```python
from build123d import *

# Parameters (mm, degrees)
SKETCH1_R               = 50
BOSS_EXTRUDE1_DEPTH     = 5
BOSS_EXTRUDE3_START     = 5
BOSS_EXTRUDE3_DEPTH     = 5
DRAFT2_ANGLE            = -45
CUT_EXTRUDE3_DEPTH      = 72.414284285
CUT_EXTRUDE3_DEPTH_BACK = 72.414284285
SKETCH3_R               = 7.5
CUT_EXTRUDE5_START      = -6.666666667
CUT_EXTRUDE5_DEPTH      = 6.666666667
SKETCH5_R               = 3.55
SKETCH5_R_2             = 1.55
CUT_EXTRUDE6_DEPTH      = 72.414284285
SKETCH5_3_R             = 3.55
SKETCH5_3_R_2           = 1.55
BOSS_EXTRUDE4_DEPTH     = 2.5
CUT_EXTRUDE8_DEPTH      = 72.414284285
CHAMFER1_SIZE           = 5
CUT_EXTRUDE9_DEPTH      = 71.887234394


with BuildPart() as part:
    # Sketch1 → Boss-Extrude1 (new body)
    with BuildSketch(Plane(origin=(0, 0, 0), x_dir=(1, 0, 0), z_dir=(0, 1, 0))):
        with Locations(Location((0, 0, 0), (0, 0, 270))):
            Circle(SKETCH1_R)
    extrude(amount=-BOSS_EXTRUDE1_DEPTH)

    # Sketch1<6> → Boss-Extrude3 (add)
    with BuildSketch(Plane(origin=(0, 0, 0), x_dir=(1, 0, 0), z_dir=(0, 1, 0)).offset(BOSS_EXTRUDE3_START)):
        with BuildLine():
            Line((-12.940952256, 48.296291314), (-34.10533906, -36.562629112))
            ThreePointArc((-34.10533906, -36.562629112), (0, -50), (34.10533906, -36.562629112))
            Line((34.10533906, -36.562629112), (12.940952256, 48.296291314))
            ThreePointArc((12.940952256, 48.296291314), (0, 50), (-12.940952256, 48.296291314))
        make_face()
    extrude(amount=-BOSS_EXTRUDE3_DEPTH)

    # Draft2
    draft2_faces = [part.faces().sort_by_distance(p)[0] for p in [
        (23.523145658, 2.5, -5.866831101),
        (-23.523145658, 2.5, -5.866831101),
    ]]
    draft(draft2_faces, Plane.ZX, DRAFT2_ANGLE)

    # Sketch3 → Cut-Extrude3 (cut, two sides: drawn at the far end of the back side and taken through both)
    with BuildSketch(Plane.XZ.offset(5).offset(-CUT_EXTRUDE3_DEPTH_BACK)):
        with Locations(Location((0, 35.355339059, 0), (0, 0, 270))):
            Circle(SKETCH3_R)
    extrude(amount=CUT_EXTRUDE3_DEPTH + CUT_EXTRUDE3_DEPTH_BACK, mode=Mode.SUBTRACT)

    # Sketch4 → Cut-Extrude5 (cut)
    with BuildSketch(Plane.XZ.offset(5).offset(CUT_EXTRUDE5_START)):
        with BuildLine():
            ThreePointArc((18.178606224, 46.578302628), (0, 50), (-18.178606224, 46.578302628))
            Line((-18.178606224, 46.578302628), (-11.548494202, 30.571796264))
            ThreePointArc((-11.548494202, 30.571796264), (3.3e-08, 22.855339059), (11.548494227, 30.571796326))
            Line((11.548494227, 30.571796326), (18.178606224, 46.578302628))
        make_face()
    extrude(amount=CUT_EXTRUDE5_DEPTH, mode=Mode.SUBTRACT)

    # Sketch5 → Cut-Extrude6 (cut, through all)
    # profile 1 of 8: a face of its own
    with BuildSketch(Plane.XZ.offset(5)):
        with Locations(Location((25.355339059, 25.355339059, 0), (0, 0, 270))):
            Circle(SKETCH5_R)
        with Locations((25.355339059, 25.355339059)):
            Circle(SKETCH5_R_2, mode=Mode.SUBTRACT)
    # profile 2 of 8: a face of its own
    with BuildSketch(Plane.XZ.offset(5)):
        with Locations((25.355339059, 25.355339059)):
            Circle(SKETCH5_R_2)
    # profile 3 of 8: a face of its own
    with BuildSketch(Plane.XZ.offset(5)):
        with Locations(Location((25.355339059, -25.355339059, 0), (0, 0, 270))):
            Circle(SKETCH5_R)
        with Locations((25.355339059, -25.355339059)):
            Circle(SKETCH5_R_2, mode=Mode.SUBTRACT)
    # profile 4 of 8: a face of its own
    with BuildSketch(Plane.XZ.offset(5)):
        with Locations((25.355339059, -25.355339059)):
            Circle(SKETCH5_R_2)
    # profile 5 of 8: a face of its own
    with BuildSketch(Plane.XZ.offset(5)):
        with Locations(Location((-25.355339059, -25.355339059, 0), (0, 0, 270))):
            Circle(SKETCH5_R)
        with Locations((-25.355339059, -25.355339059)):
            Circle(SKETCH5_R_2, mode=Mode.SUBTRACT)
    # profile 6 of 8: a face of its own
    with BuildSketch(Plane.XZ.offset(5)):
        with Locations((-25.355339059, -25.355339059)):
            Circle(SKETCH5_R_2)
    # profile 7 of 8: a face of its own
    with BuildSketch(Plane.XZ.offset(5)):
        with Locations(Location((-25.355339059, 25.355339059, 0), (0, 0, 270))):
            Circle(SKETCH5_R)
        with Locations((-25.355339059, 25.355339059)):
            Circle(SKETCH5_R_2, mode=Mode.SUBTRACT)
    # profile 8 of 8: a face of its own
    with BuildSketch(Plane.XZ.offset(5)):
        with Locations((-25.355339059, 25.355339059)):
            Circle(SKETCH5_R_2)
    extrude(amount=-CUT_EXTRUDE6_DEPTH, mode=Mode.SUBTRACT)

    # Sketch5<3> → Boss-Extrude4 (add)
    # profile 1 of 4: a face of its own
    with BuildSketch(Plane.XZ.offset(5)):
        with Locations(Location((25.355339059, -25.355339059, 0), (0, 0, 270))):
            Circle(SKETCH5_3_R)
        with Locations(Location((25.355339059, -25.355339059, 0), (0, 0, 270))):
            Circle(SKETCH5_3_R_2, mode=Mode.SUBTRACT)
    # profile 2 of 4: a face of its own
    with BuildSketch(Plane.XZ.offset(5)):
        with Locations(Location((-25.355339059, -25.355339059, 0), (0, 0, 270))):
            Circle(SKETCH5_3_R)
        with Locations(Location((-25.355339059, -25.355339059, 0), (0, 0, 270))):
            Circle(SKETCH5_3_R_2, mode=Mode.SUBTRACT)
    # profile 3 of 4: a face of its own
    with BuildSketch(Plane.XZ.offset(5)):
        with Locations(Location((25.355339059, 25.355339059, 0), (0, 0, 270))):
            Circle(SKETCH5_3_R)
        with Locations(Location((25.355339059, 25.355339059, 0), (0, 0, 270))):
            Circle(SKETCH5_3_R_2, mode=Mode.SUBTRACT)
    # profile 4 of 4: a face of its own
    with BuildSketch(Plane.XZ.offset(5)):
        with Locations(Location((-25.355339059, 25.355339059, 0), (0, 0, 270))):
            Circle(SKETCH5_3_R)
        with Locations(Location((-25.355339059, 25.355339059, 0), (0, 0, 270))):
            Circle(SKETCH5_3_R_2, mode=Mode.SUBTRACT)
    extrude(amount=-BOSS_EXTRUDE4_DEPTH)

    # Sketch6 → Cut-Extrude8 (cut, through all)
    with BuildSketch(Plane(origin=(0, 5, 0), x_dir=(1, 0, 0), z_dir=(0, 1, 0))):
        with BuildLine():
            ThreePointArc((-0.574925376, -22.523405739), (0, -22.191472419), (0.574925376, -22.523405739))
            Line((0.574925376, -22.523405739), (19.793304237, -11.42766953))
            Line((19.793304237, -11.42766953), (19.793304237, 11.42766953))
            Line((19.793304237, 11.42766953), (0, 22.855339059))
            Line((0, 22.855339059), (-19.793304237, 11.42766953))
            Line((-19.793304237, 11.42766953), (-19.793304237, -11.42766953))
            Line((-19.793304237, -11.42766953), (-0.574925376, -22.523405739))
        make_face()
    extrude(amount=-CUT_EXTRUDE8_DEPTH, mode=Mode.SUBTRACT)

    # Chamfer1
    chamfer1_edges = [part.edges().sort_by_distance(p)[0] for p in [
        (-25.355339059, 5, 28.905339059),
        (25.355339059, 5, 28.905339059),
    ]]
    chamfer(chamfer1_edges, length=CHAMFER1_SIZE)

    # Sketch7 → Cut-Extrude9 (cut, symmetric)
    with BuildSketch(Plane(origin=(0, 0, 0), x_dir=(1, 0, 0), z_dir=(0, 1, 0))):
        with BuildLine():
            ThreePointArc((-34.768601784, 26.965613845), (-43.954325541, 2.004311919), (-37.078464111, -23.689396344))
            Line((-37.078464111, -23.689396344), (-27.184130942, 15.982078141))
            ThreePointArc((-27.184130942, 15.982078141), (-33.213803419, 19.928826559), (-34.768601784, 26.965613845))
        make_face()
    cut_extrude9 = extrude(amount=CUT_EXTRUDE9_DEPTH, both=True, mode=Mode.SUBTRACT)

    # Mirror1: Cut-Extrude9 across plane
    add(cut_extrude9.mirror(Plane(origin=(0, 0, 0), x_dir=(0, 0, 1), z_dir=(1, 0, 0))), mode=Mode.SUBTRACT)


solid = part.part
```
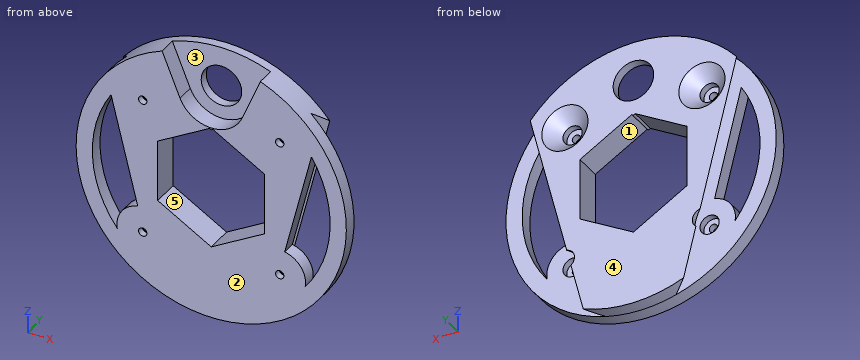
Read the model definition and answer for the solid it produces. Units are mm, in the model's axes. Face numbers are marked on the shaded views. A direction names the side the tool comes from. Coordinates: 2 decimals unless noted, no trailing zeros. Write each loop counter-clockwise with the first axis right and the second up, starting at its lowest first coordinate (ties: lowest second). Pieces come first, ordered by that corner, then holes. Notation, with made-up numbers: (87.5, 16) - (135.5, 16) arc R13 cw to (135.5, 27) - close; hole circle Ø9 at (82.5, 61). An arc over 180 degrees is marked (long way). Answer as a JSON object with one key per item and string values. Group by question number.
1. A cutting plane is placed at B-B (z = 0). Determine the outline of the cut face in (x, y).
2. Consider L1, parallel to X at y = -0.5, z = -2; L2, parallel to X at y = -1.5, z = -9; L3, parallel to X at y = 0.5, z = -17. Determine where each line is inside the solid, lowest interval first. Write a range as [from, to].
3. A cutting plane is placed at D-D (z = 39.5). Determine the outline of the cut face in (x, y).
4. A cutting plane is placed at A-A (x = -41). Determine the outline of the cut face in (y, z), plus the area to 3 significant figures.
5. The mould has two halves that part along X. Classify the marked faces 1 and 2: +X half, -X half, draft (parallel to the pull), parting line (faces both ways), or undercut.
6. Each of these flat-tipped pins is pushed along its axis until it touches: P1, Ø9, axis at x = -25.36, z = -25.36, coming from the -Y side; P2, Ø8, axis at x = -26, z = 25, coming from the +Y side; P3, Ø3, axis at x = 16.5, z = -1.5, coming from the -Y side; P4, Ø3.5, axis at x = 27, z = 25.5, coming from the +Y side. Where does it stop, or does it pass through?
7. Which of the six approach directions +Z, -Z, +X, -X, +Y, -Y give full straight-line access (tool end or side, diameter ignored) to the marked faces 3, 4 and 5?
8. A cutting plane is placed at C-C (x = 3.5). Determine the outline of the cut face in (y, z), plus the area to 3 significant figures.
Worked out:
{
 "1": {"outline": "(-50, -5) - (-44, -5) - (-44, 0) - (-50, 0) - close; (-31.17, -5) - (-19.79, -5) - (-19.79, 5) - (-30.14, 5) - (-24.99, 0) - (-31.17, 0) - close; (19.79, -5) - (31.17, -5) - (31.17, 0) - (24.99, 0) - (30.14, 5) - (19.79, 5) - close; (44, -5) - (50, -5) - (50, 0) - (44, 0) - close"},
 "2": {"L1": "x = [-49.96, -43.95], [-30.67, -19.79], [19.79, 30.67], [43.95, 49.96]", "L2": "x = [-49.18, -43.07], [-28.93, -19.79], [19.79, 28.93], [43.07, 49.18]", "L3": "x = [-21.26, -10.14], [10.14, 21.26]"},
 "3": {"outline": "(-30.66, -5) - (-15.25, -5) - (-15.25, 1.67) - (-6.25, 1.67) - (-6.25, 5) - (-30.66, 5) - close; (6.25, 1.67) - (15.25, 1.67) - (15.25, -5) - (30.66, -5) - (30.66, 5) - (6.25, 5) - close"},
 "4": {"outline": "(-5, -28.62) - (0, -28.62) - (0, -15.97) - (-5, -15.97) - close; (-5, 15.97) - (0, 15.97) - (0, 28.62) - (-5, 28.62) - close", "area": "126 mm²"},
 "5": {"face 1": "undercut", "face 2": "draft"},
 "6": {"P1": "stops at y = -5", "P2": "stops at y = 1.19", "P3": "passes through", "P4": "stops at y = -2.5"},
 "7": {"face 3": "+Z, -Y", "face 4": "+Z, -Z, +X, -X, +Y", "face 5": "+Y, -Y"},
 "8": {"outline": "(-5, -49.88) - (5, -49.88) - (5, -20.83) - (-5, -20.83) - close; (-5, 20.83) - (5, 20.83) - (5, 28.72) - (1.67, 28.72) - (1.67, 23.36) - (-5, 23.36) - close; (1.67, 41.99) - (5, 41.99) - (5, 49.88) - (1.67, 49.88) - close", "area": "360 mm²"}
}
